Source: CAD feature listing. Evaluate the final solid. Frame: model axes, mm. A direction names the side the tool comes from. Give positions to 0.01 mm unless a question says otherwise; leave off trailing zeros. Write each loop counter-clockwise with the first axis right and the second up, starting at its lowest first coordinate (ties: lowest second). Pieces come first, ordered by that corner, then holes. Notation, with made-up numbers: (55.25, 34) - (69.25, 34) arc R3 cw to (69.25, 39) - close; hole circle Ø7 at (60.5, 11.5). An arc over 180 degrees is marked (long way). One line per question, with ' | ' between items. Start each with the question number.
(1) Section A-A, the plane x = 0. Return loops of the section in (y, z).
(2) Pin query (flat end, axial travel): pin 1 (3 mm diameter, centred on y = -20, z = 19, fed in from +X); pin 2 (12.5 mm diameter, centred on x = -4, z = 21.5, fed in from +Y); pin 3 (6 mm diameter, centred on x = 5, y = -4, fed in from +Z). Return the tip coordinate at first contact, or that it passes through.
(3) Draft query along Z for faces 1 (the flat face through (-0.03, -14.06, 6.99)), 2 (the flat face through (0, -23, 4.8)), 3 (the cylindrical face through (-12.658, -12.038, 4.187)). Return one class per face: +Z half, -Z half, draft (parallel to the pull), parting line (faces both ways), or undercut.
(4) Section D-D, the plane y = -10. Return loops of the section in (x, z), plus the area to 3 significant figures.
(5) Section B-B, the plane y = 10. Return loops of the section in (x, z), plus the area to 3 significant figures.
(6) Section C-C, the plane x = -10. Return loops of the section in (y, z).
(7) Access query for faces 4 (the flat face through (-12.7, -20, 14)), 5 (the cylindrical face through (9.27, -13.27, 4.19)), 6 (the flat face through (0, -20, 5)). Directions: +Z, -Z, +X, -X, +Y, -Y. A direction counts if a zero-diameter tool reaches every point of the face in a straight line with its end or side. Return the directions, or none.
(8) Ray query, line 1 (Y direction, x = -10, z = 4.6); line 2 (Y direction, x = 10, z = 1.95); line 3 (Y direction, x = 0, z = 2.7). Return the intervals inside material, ascending. Write a range as [from, to].
```python
from build123d import *

# Parameters (mm, degrees)
SKETCH1_W                       = 30
SKETCH1_H                       = 32
BOSS_EXTRUDE1_DEPTH             = 5
CBORE_FOR_M3_SBHCS2_D           = 3.4
CBORE_FOR_M3_SBHCS2_CBORE_D     = 6.7
CBORE_FOR_M3_SBHCS2_CBORE_DEPTH = 1.65
TAP_DRILL_FOR_M3X0_5_TAP1_D     = 2.5
SKETCH5_W                       = 25.4
SKETCH5_H                       = 30.4
BOSS_EXTRUDE2_DEPTH             = 5
BOSS_EXTRUDE3_REACH             = 38.377
SKETCH8_W                       = 5
SKETCH8_H                       = 10
BOSS_EXTRUDE3_DIRECTION_2_REACH = 38.377
SKETCH10_W                      = 6.6
SKETCH10_H                      = 19.4
CUT_EXTRUDE1_DEPTH              = 2.7
FILLET1_R                       = 1
SKETCH12_W                      = 25.4
SKETCH12_H                      = 4.8
BOSS_EXTRUDE5_DEPTH             = 5
FILLET2_START                   = -1
FILLET2_DEPTH                   = 30.4
FILLET2_2_DEPTH                 = 5


with BuildPart() as part:
    # Sketch1 → Boss-Extrude1 (new body)
    with BuildSketch(Plane.XY):
        Rectangle(SKETCH1_W, SKETCH1_H)
    extrude(amount=BOSS_EXTRUDE1_DEPTH)

    # CBORE for M3 SBHCS2 (through all)
    with Locations(Plane.XY.offset(5)):
        with Locations((-10, 10), (-10, -10), (10, -10), (10, 10)):
            CounterBoreHole(CBORE_FOR_M3_SBHCS2_D / 2, CBORE_FOR_M3_SBHCS2_CBORE_D / 2, CBORE_FOR_M3_SBHCS2_CBORE_DEPTH)

    # Tap Drill for M3x0.5 Tap1 (through all)
    with Locations(Plane.XY.offset(5)):
        with Locations((0, 10)):
            Hole(TAP_DRILL_FOR_M3X0_5_TAP1_D / 2)

    # Sketch5 → Boss-Extrude2 (add)
    with BuildSketch(Plane.XZ.offset(16)):
        with Locations((0, 15.2)):
            Rectangle(SKETCH5_W, SKETCH5_H)
    extrude(amount=BOSS_EXTRUDE2_DEPTH)

    # Boss-Extrude3: up to this plane
    boss_extrude3_end = Plane(origin=(0, -16, 0), z_dir=(0, -1, 0))
    # Sketch8 → Boss-Extrude3 (add, up to the surface)
    with BuildSketch(Plane(origin=(0, -10.5, 10.5), x_dir=(1, 0, 0), z_dir=(0, -0.7071067811865475, 0.7071067811865477)), mode=Mode.PRIVATE) as boss_extrude3_sk1:
        Rectangle(SKETCH8_W, SKETCH8_H)
    boss_extrude3_tool1 = split(extrude(boss_extrude3_sk1.sketch, amount=BOSS_EXTRUDE3_REACH, mode=Mode.PRIVATE), bisect_by=boss_extrude3_end, keep=Keep.BOTH, mode=Mode.PRIVATE)
    add(boss_extrude3_tool1.solids().sort_by_distance((0, -10.5, 10.5))[0])

    # Boss-Extrude3 direction 2: up to this plane
    boss_extrude3_direction_2_end = Plane(origin=(0, 0, 5), z_dir=(0, 0, 1))
    # Sketch8 → Boss-Extrude3 direction 2 (add, up to the surface)
    with BuildSketch(Plane(origin=(0, -10.5, 10.5), x_dir=(1, 0, 0), z_dir=(0, -0.7071067811865475, 0.7071067811865477)), mode=Mode.PRIVATE) as boss_extrude3_direction_2_sk1:
        Rectangle(SKETCH8_W, SKETCH8_H)
    boss_extrude3_direction_2_tool1 = split(extrude(boss_extrude3_direction_2_sk1.sketch, amount=-BOSS_EXTRUDE3_DIRECTION_2_REACH, mode=Mode.PRIVATE), bisect_by=boss_extrude3_direction_2_end, keep=Keep.BOTH, mode=Mode.PRIVATE)
    add(boss_extrude3_direction_2_tool1.solids().sort_by_distance((0, -10.5, 10.5))[0])

    # Sketch10 → Cut-Extrude1 (cut)
    with BuildSketch(Plane.XZ.offset(21)):
        with Locations((0, 14.7)):
            Rectangle(SKETCH10_W, SKETCH10_H)
    extrude(amount=-CUT_EXTRUDE1_DEPTH, mode=Mode.SUBTRACT)

    # Fillet1
    fillet1_edges = [part.edges().sort_by_distance(p)[0] for p in [
        (12.7, -18.5, 30.4),
        (-12.7, -18.5, 30.4),
    ]]
    fillet(fillet1_edges, radius=FILLET1_R)

    # Sketch12 → Boss-Extrude5 (add)
    with BuildSketch(Plane.XZ.offset(21)):
        with Locations((0, 2.4)):
            Rectangle(SKETCH12_W, SKETCH12_H)
    extrude(amount=BOSS_EXTRUDE5_DEPTH)

    # Fillet2: read off the stored shape, not the designer's step
    # Fillet2 outline → Fillet2 (cut)
    with BuildSketch(Plane.XY.offset(FILLET2_START)):
        with BuildLine():
            Line((15, -16), (15, -14.9))
            ThreePointArc((15, -14.9), (14.677817459, -15.677817459), (13.9, -16))
            Line((13.9, -16), (15, -16))
        make_face()
        with BuildLine():
            Line((-15, -16), (-13.9, -16))
            ThreePointArc((-13.9, -16), (-14.677817459, -15.677817459), (-15, -14.9))
            Line((-15, -14.9), (-15, -16))
        make_face()
    extrude(amount=FILLET2_DEPTH, mode=Mode.SUBTRACT)

    # Fillet2 2 outline → Fillet2 2 (add)
    with BuildSketch(Plane.XY):
        with BuildLine():
            ThreePointArc((12.7, -17.1), (13.022182541, -16.322182541), (13.8, -16))
            Line((13.8, -16), (12.7, -16))
            Line((12.7, -16), (12.7, -17.1))
        make_face()
        with BuildLine():
            Line((-12.7, -16), (-13.8, -16))
            ThreePointArc((-13.8, -16), (-13.022182541, -16.322182541), (-12.7, -17.1))
            Line((-12.7, -17.1), (-12.7, -16))
        make_face()
    extrude(amount=FILLET2_2_DEPTH)


solid = part.part
```
Check sheet entries:
1) outline: (-26, 0) - (8.75, 0) - (8.75, 5) - (2.07, 5) - (-16, 23.07) - (-16, 30.4) - (-21, 30.4) - (-21, 24.4) - (-18.3, 24.4) - (-18.3, 5) - (-21, 5) - (-21, 4.8) - (-26, 4.8) - close; (11.25, 0) - (16, 0) - (16, 5) - (11.25, 5) - close; hole (-16, 5) - (-12.07, 5) - (-16, 8.93) - close
2) pin 1: x = 12.7 | pin 2: y = -8.36 | pin 3: z = 12.73
3) face 1: undercut | face 2: +Z half | face 3: draft
4) outline: (-15, 0) - (-11.7, 0) - (-11.7, 3.35) - (-13.35, 3.35) - (-13.35, 5) - (-15, 5) - close; (-8.3, 0) - (8.3, 0) - (8.3, 3.35) - (6.65, 3.35) - (6.65, 5) - (2.5, 5) - (2.5, 17.07) - (-2.5, 17.07) - (-2.5, 5) - (-6.65, 5) - (-6.65, 3.35) - (-8.3, 3.35) - close; (11.7, 0) - (15, 0) - (15, 5) - (13.35, 5) - (13.35, 3.35) - (11.7, 3.35) - close | area: 165 mm²
5) outline: (-15, 0) - (-11.7, 0) - (-11.7, 3.35) - (-13.35, 3.35) - (-13.35, 5) - (-15, 5) - close; (-8.3, 0) - (-1.25, 0) - (-1.25, 5) - (-6.65, 5) - (-6.65, 3.35) - (-8.3, 3.35) - close; (1.25, 0) - (8.3, 0) - (8.3, 3.35) - (6.65, 3.35) - (6.65, 5) - (1.25, 5) - close; (11.7, 0) - (15, 0) - (15, 5) - (13.35, 5) - (13.35, 3.35) - (11.7, 3.35) - close | area: 92.6 mm²
6) outline: (-26, 0) - (-11.7, 0) - (-11.7, 3.35) - (-13.35, 3.35) - (-13.35, 5) - (-16, 5) - (-16, 30.4) - (-21, 30.4) - (-21, 4.8) - (-26, 4.8) - close; (-8.3, 0) - (8.3, 0) - (8.3, 3.35) - (6.65, 3.35) - (6.65, 5) - (-6.65, 5) - (-6.65, 3.35) - (-8.3, 3.35) - close; (11.7, 0) - (16, 0) - (16, 5) - (13.35, 5) - (13.35, 3.35) - (11.7, 3.35) - close
7) face 4: +Z, -X, -Y | face 5: +Z | face 6: -Y
8) line 1: [-26, -13.35], [-6.65, 6.65], [13.35, 16] | line 2: [-26, -11.7], [-8.3, 8.3], [11.7, 16] | line 3: [-26, 8.75], [11.25, 16]
